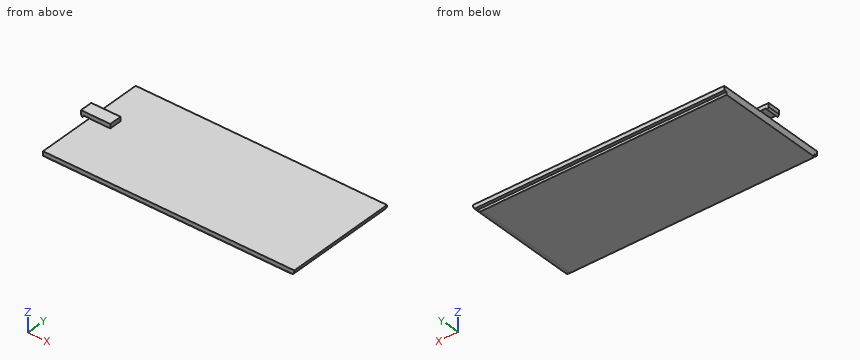
```python
from build123d import *

# Parameters (mm, degrees)
SKETCH1_W           = 180
SKETCH1_H           = 81
BOSS_EXTRUDE1_DEPTH = 5
FILLET1_R           = 5
SKETCH2_W           = 2
SKETCH2_H           = 2
CUT_EXTRUDE1_DEPTH  = 185.567738243
SKETCH3_W           = 15
SKETCH3_H           = 9
BOSS_EXTRUDE2_DEPTH = 3
SKETCH4_W           = 2.8
SKETCH4_H           = 9
BOSS_EXTRUDE3_DEPTH = 6
BOSS_EXTRUDE4_DEPTH = 9


with BuildPart() as part:
    # Sketch1 → Boss-Extrude1 (new body)
    with BuildSketch(Plane.XY):
        Rectangle(SKETCH1_W, SKETCH1_H)
    extrude(amount=BOSS_EXTRUDE1_DEPTH)

    # Fillet1
    fillet1_edges = [part.edges().sort_by_distance(p)[0] for p in [
        (90, 0, 0),
    ]]
    fillet(fillet1_edges, radius=FILLET1_R - 0.0001)  # a hair under: the kernel refuses the full size

    # Sketch2 → Cut-Extrude1 (cut, through all)
    with BuildSketch(Plane.ZY.offset(90)):
        with Locations((1, 39.5)):
            Rectangle(SKETCH2_W, SKETCH2_H)
        with Locations((1, -39.5)):
            Rectangle(SKETCH2_W, SKETCH2_H)
    extrude(amount=-CUT_EXTRUDE1_DEPTH, mode=Mode.SUBTRACT)

    # Sketch3 → Boss-Extrude2 (add)
    with BuildSketch(Plane.XY.offset(5)):
        with Locations((-82.5, 4.5)):
            Rectangle(SKETCH3_W, SKETCH3_H)
    extrude(amount=BOSS_EXTRUDE2_DEPTH)

    # Sketch4 → Boss-Extrude3 (add)
    with BuildSketch(Plane.ZY.offset(90)):
        with Locations((6.6, 4.5)):
            Rectangle(SKETCH4_W, SKETCH4_H)
    extrude(amount=BOSS_EXTRUDE3_DEPTH)

    # Sketch5 → Boss-Extrude4 (add)
    with BuildSketch(Plane(origin=(0, 9, 0), x_dir=(1, 0, 0), z_dir=(0, 1, 0))):
        Polygon((-96, -5.2), (-95.031000632, -3.7), (-94, -5.2), align=None)
    extrude(amount=-BOSS_EXTRUDE4_DEPTH)


solid = part.part
```
Can you work these out from the model? Positions are in its coordinate system, mm. Give positions to 0.01 mm unless a question says otherwise; leave off trailing zeros. Loops run counter-clockwise (first coordinate to the right, second up) from the corner with the lowest first, then second, coordinate; pieces in that order, holes last. Notation, with made-up numbers: M 28,45.5 L 58,45.5 A14 cw 58,67.5 Z; hole C 81,18 d5. An arc over 180 degrees is marked long. One line per question, with ' | ' between items. Start each with the question number.
Q1. If we section it at A-A (x = -6): Please give me the cut outline in (y, z), plus the area to 3 significant figures.
Q2. For pin 1 Ø12 at (x, y) = (49.5, -3.5) entering from +Z; pin 2 Ø2.5 at (y, z) = (4.5, 6) entering from +X; pin 3 Ø0.6 at (x, y) = (15.5, 39) entering from -Z; pin 4 Ø1.3 at (x, z) = (-83, 6.5) entering from -Y, each with a flat end and sliding along its axis, tell me the tip position at first contact or that it passes through.
Q3. If I drill on line 1 (Z direction, x = 25, y = 16); line 2 (X direction, y = 29, z = 2); line 3 (Y direction, x = 21, z = 1.25), over which ranges is the centre line in solid material (lowest first)? Write a range as from..to.
Computed:
1) outline: M -40.5,2 L -38.5,2 L -38.5,0 L 38.5,0 L 38.5,2 L 40.5,2 L 40.5,5 L -40.5,5 Z | area: 397 mm²
2) pin 1: stops at z = 5 | pin 2: stops at x = 90 | pin 3: stops at z = 2 | pin 4: stops at y = 0
3) line 1: z = 0..5 | line 2: x = -90..89 | line 3: y = -38.5..38.5
